Design review of the part built by this model. Coordinates are the model's own, in mm. Round coordinates to 2 decimals unless told otherwise and drop trailing zeros. Order: outer loops, then holes, each group sorted by start corner. A loop starts at its lowest first (then second) coordinate and runs counter-clockwise, first axis right, second up. Notation, with made-up numbers: M 30.5,-0.5 L 48.5,-0.5 A30 ccw 48.5,23.5 Z; hole C 56.25,82.25 d3. An arc over 180 degrees is marked long. Write each question's results on one line, items separated by ' | '. Start each with the question number.
Item 1: The part is to be moulded in two halves that separate along Y. For faces 1 (the flat face through (13, 0, 0)), 2 (the cylindrical face through (7.605, 13.163, -5.458)), 3 (the cylindrical face through (7.6, 5.19, -9.98)), 4 (the flat face through (0, 11, -4)), say which applies: +Y half, -Y half, draft (parallel to the pull), parting line (faces both ways), or undercut.
Item 2: Take a section at A-A, the plane x = 6. Write out the cut boundary in (y, z).
Item 3: Clearance check with flat-ended pins moving along their axes: pin 1 (12 mm diameter, centred on y = 9.5, z = -7, fed in from +X); pin 2 (10 mm diameter, centred on x = 8, z = 8, fed in from -Y); pin 3 (2.5 mm diameter, centred on y = 0, z = 0.5, fed in from -X). State where each tip first meets the part, or that it passes through.
Item 4: Wall thickness on line 1 (Z direction, x = 14.75, y = 0); line 2 (Y direction, x = 2, z = -10.25); line 3 (Z direction, x = 14, y = 1.5): over which ranges is each line inside the solid? List them lowest first. Write a range as [from, to].
```python
from build123d import *

# Parameters (mm, degrees)
F0_W     = 15
F0_H     = 3
F2_R     = 4.1
F4_R     = 4
F5_DEPTH = 13


with BuildPart() as f1:
    # F0 (on Top) → F1 (revolve)
    with BuildSketch(Plane.XY):
        with BuildLine():
            Line((15, 14.25), (15, 11.25))
            ThreePointArc((15, 11.25), (16.2836091475, 5.6846908501), (16.8355224703, 0))
            Line((16.8355224703, 0), (17.9961773834, 0))
            ThreePointArc((17.9961773834, 0), (17.2938882179, 7.2923232661), (15, 14.25))
        make_face()
        with Locations((7.5, 12.75)):
            Rectangle(F0_W, F0_H)
    revolve(axis=Axis((8.9980886917, 0, 0), (1, 0, 0)))

    # F2 (on Right) → F3 (join, up to the next surface of F1)
    with BuildSketch(Plane.YZ):
        Circle(F2_R)
    extrude(until=Until.NEXT)

    # F4 (on face) → F5 (cut)
    with BuildSketch(Plane(origin=(0, 0, 0), x_dir=(0, -1, 0), z_dir=(-1, 0, 0))):
        Circle(F4_R)
    extrude(amount=-F5_DEPTH, mode=Mode.SUBTRACT)


solid = f1.part
```
Results list:
1) face 1: undercut | face 2: parting line | face 3: undercut | face 4: draft
2) outline: C 0,0 d28.5; C 0,0 d8.2; hole C 0,0 d22.5; hole C 0,0 d8
3) pin 1: x = 17.57 | pin 2: y = -13.93 | pin 3: x = 13
4) line 1: [-14.25, -11.25], [-4.1, 4.1], [11.25, 14.25] | line 2: [-9.9, -4.64], [4.64, 9.9] | line 3: [-14.17, -11.15], [-3.82, 3.82], [11.15, 14.17]
